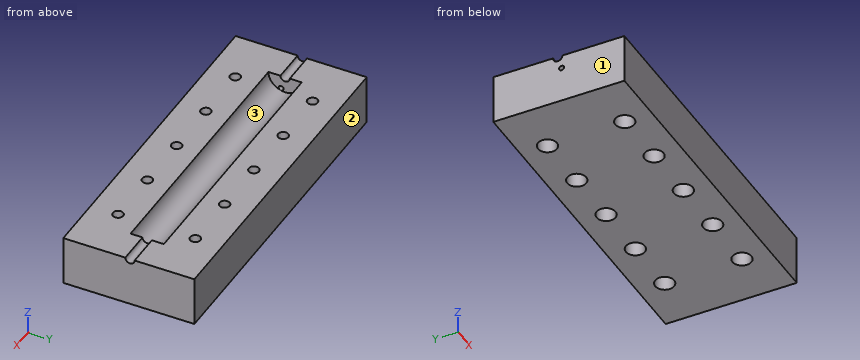
from build123d import *

# Parameters (mm, degrees)
SKIZZE2_W                            = 100
SKIZZE2_H                            = 39.364160046
AUFSATZ_LINEAR_AUSTRAGEN1_DEPTH      = 30
SCHNITT_LINEAR_AUSTRAGEN1_DEPTH      = 40
SCHNITT_LINEAR_AUSTRAGEN1_DEPTH_BACK = 40
SKIZZE10_R                           = 5
SKIZZE17_R                           = 1.4
SCHNITT_LINEAR_AUSTRAGEN2_DEPTH      = 103.710939516
SKIZZE24_R                           = 1.55
SCHNITT_LINEAR_AUSTRAGEN4_DEPTH      = 112.577493681
SKIZZE37_R                           = 0.736865544
SCHNITT_LINEAR_AUSTRAGEN9_DEPTH      = 112.577493681
SKIZZE40_R                           = 2.1
SCHNITT_LINEAR_AUSTRAGEN10_DEPTH     = 6
SKIZZE42_R                           = 0.75
SCHNITT_LINEAR_AUSTRAGEN12_DEPTH     = 10
VERRUNDUNG1_R                        = 1
SKIZZE46_R                           = 2.85
SCHNITT_LINEAR_AUSTRAGEN15_DEPTH     = 10
SCHNITT_LINEAR_START                 = -5
SCHNITT_LINEAR_AUSTRAGEN25_DEPTH     = 2.7
LINEARES_MUSTER1_COUNT               = 5
LINEARES_MUSTER1_PITCH               = 17
SPIEGELN2_COPY_1_SKETCH_R            = 2.85
SPIEGELN2_COPY_1_DEPTH               = 10
SPIEGELN2_COPY_2_SKETCH_R            = 2.85
SPIEGELN2_COPY_2_DEPTH               = 10
SPIEGELN2_COPY_3_SKETCH_R            = 2.85
SPIEGELN2_COPY_3_DEPTH               = 10
SPIEGELN2_COPY_4_SKETCH_R            = 2.85
SPIEGELN2_COPY_4_DEPTH               = 10
SPIEGELN2_START                      = -5
SPIEGELN2_COPY_5_DEPTH               = 2.7
SPIEGELN2_COPY_6_DEPTH               = 2.7
SPIEGELN2_COPY_7_DEPTH               = 2.7
SPIEGELN2_COPY_8_DEPTH               = 2.7
SKIZZE51_W                           = 15
SKIZZE51_H                           = 39.364160046
SCHNITT_LINEAR_AUSTRAGEN26_DEPTH     = 112.577493681


with BuildPart() as part:
    # Skizze2 → Aufsatz-Linear austragen1 (new body)
    with BuildSketch(Plane.XY):
        with Locations((50, 19.682080023)):
            Rectangle(SKIZZE2_W, SKIZZE2_H)
    extrude(amount=AUFSATZ_LINEAR_AUSTRAGEN1_DEPTH)

    # Skizze10 → Schnitt-Linear austragen1 (cut, two sides: drawn at the far end of the back side and taken through both)
    with BuildSketch(Plane.ZY.offset(-50).offset(-SCHNITT_LINEAR_AUSTRAGEN1_DEPTH_BACK)):
        with Locations((14.945770016, 20.027045739)):
            Circle(SKIZZE10_R)
    extrude(amount=SCHNITT_LINEAR_AUSTRAGEN1_DEPTH + SCHNITT_LINEAR_AUSTRAGEN1_DEPTH_BACK, mode=Mode.SUBTRACT)

    # Skizze17 → Schnitt-Linear austragen2 (cut, through all)
    with BuildSketch(Plane.ZY.offset(-90)):
        with Locations((14.945770016, 20.027045739)):
            Circle(SKIZZE17_R)
    schnitt_linear_austragen2 = extrude(amount=-SCHNITT_LINEAR_AUSTRAGEN2_DEPTH, mode=Mode.SUBTRACT)

    # Spiegeln1: Schnitt-Linear austragen2 across plane
    add(schnitt_linear_austragen2.mirror(Plane.ZY.offset(-50)), mode=Mode.SUBTRACT)

    # Skizze24 → Schnitt-Linear austragen4 (cut, through all)
    with BuildSketch(Plane.XY.offset(30)):
        with Locations((16, 31.364160046)):
            Circle(SKIZZE24_R)
        with Locations((33, 31.364160046)):
            Circle(SKIZZE24_R)
        with Locations((50, 31.364160046)):
            Circle(SKIZZE24_R)
        with Locations((67, 31.364160046)):
            Circle(SKIZZE24_R)
        with Locations((84, 31.364160046)):
            Circle(SKIZZE24_R)
    schnitt_linear_austragen4 = extrude(amount=-SCHNITT_LINEAR_AUSTRAGEN4_DEPTH, mode=Mode.SUBTRACT)

    # Skizze37 → Schnitt-Linear austragen9 (cut, through all)
    with BuildSketch(Plane(origin=(100, 0, 0), x_dir=(0, 0, -1), z_dir=(1, 0, 0))):
        with Locations((-18.924590299, 18.633559666)):
            Circle(SKIZZE37_R)
    extrude(amount=-SCHNITT_LINEAR_AUSTRAGEN9_DEPTH, mode=Mode.SUBTRACT)

    # Skizze40 → Schnitt-Linear austragen10 (cut)
    with BuildSketch(Plane(origin=(100, 0, 0), x_dir=(0, 0, -1), z_dir=(1, 0, 0))):
        with Locations((-18.924590299, 18.633559666)):
            Circle(SKIZZE40_R)
    extrude(amount=-SCHNITT_LINEAR_AUSTRAGEN10_DEPTH, mode=Mode.SUBTRACT)

    # Skizze42 → Schnitt-Linear austragen12 (cut)
    with BuildSketch(Plane.ZY):
        with Locations((10.86415918, 18.842582577)):
            Circle(SKIZZE42_R)
    extrude(amount=-SCHNITT_LINEAR_AUSTRAGEN12_DEPTH, mode=Mode.SUBTRACT)

    # Verrundung1
    verrundung1_edges = [part.edges().sort_by_distance(p)[0] for p in [
        (94, 18.633559666, 19.661455843),
    ]]
    fillet(verrundung1_edges, radius=VERRUNDUNG1_R)

    # Skizze46 → Schnitt-Linear austragen15 (cut)
    with BuildSketch(Plane(origin=(0, 0, 0), x_dir=(-1, 0, 0), z_dir=(0, 0, -1))):
        with Locations((-84, 31.364160046)):
            Circle(SKIZZE46_R)
    schnitt_linear_austragen15 = extrude(amount=-SCHNITT_LINEAR_AUSTRAGEN15_DEPTH, mode=Mode.SUBTRACT)

    # Skizze50 → Schnitt-Linear austragen25 (cut)
    with BuildSketch(Plane.XY.offset(30).offset(SCHNITT_LINEAR_START)):
        Polygon((81.15, 33.009608314), (81.15, 39.364160046), (86.85, 39.364160046), (86.85, 33.009608314), (86.85, 29.718711779), (84, 28.073263512), (81.15, 29.718711779), align=None)
    schnitt_linear_austragen25 = extrude(amount=-SCHNITT_LINEAR_AUSTRAGEN25_DEPTH, mode=Mode.SUBTRACT)

    # Lineares Muster1: Schnitt-Linear austragen15, Schnitt-Linear austragen25 ×5
    with Locations(*[(-i * LINEARES_MUSTER1_PITCH, 0, 0) for i in range(1, LINEARES_MUSTER1_COUNT)]):
        add(schnitt_linear_austragen15, mode=Mode.SUBTRACT)
        add(schnitt_linear_austragen25, mode=Mode.SUBTRACT)

    # Spiegeln2: Schnitt-Linear austragen15, Schnitt-Linear austragen25 across plane
    add(schnitt_linear_austragen15.mirror(Plane.ZX.offset(19.764160046)), mode=Mode.SUBTRACT)
    add(schnitt_linear_austragen25.mirror(Plane.ZX.offset(19.764160046)), mode=Mode.SUBTRACT)

    # Spiegeln2 copy 1 sketch → Spiegeln2 copy 1 (cut)
    with BuildSketch(Plane(origin=(-17, 39.528320093, 0), x_dir=(-1, 0, 0), z_dir=(0, 0, -1))):
        with Locations((-84, -31.364160046)):
            Circle(SPIEGELN2_COPY_1_SKETCH_R)
    extrude(amount=-SPIEGELN2_COPY_1_DEPTH, mode=Mode.SUBTRACT)

    # Spiegeln2 copy 2 sketch → Spiegeln2 copy 2 (cut)
    with BuildSketch(Plane(origin=(-34, 39.528320093, 0), x_dir=(-1, 0, 0), z_dir=(0, 0, -1))):
        with Locations((-84, -31.364160046)):
            Circle(SPIEGELN2_COPY_2_SKETCH_R)
    extrude(amount=-SPIEGELN2_COPY_2_DEPTH, mode=Mode.SUBTRACT)

    # Spiegeln2 copy 3 sketch → Spiegeln2 copy 3 (cut)
    with BuildSketch(Plane(origin=(-51, 39.528320093, 0), x_dir=(-1, 0, 0), z_dir=(0, 0, -1))):
        with Locations((-84, -31.364160046)):
            Circle(SPIEGELN2_COPY_3_SKETCH_R)
    extrude(amount=-SPIEGELN2_COPY_3_DEPTH, mode=Mode.SUBTRACT)

    # Spiegeln2 copy 4 sketch → Spiegeln2 copy 4 (cut)
    with BuildSketch(Plane(origin=(-68, 39.528320093, 0), x_dir=(-1, 0, 0), z_dir=(0, 0, -1))):
        with Locations((-84, -31.364160046)):
            Circle(SPIEGELN2_COPY_4_SKETCH_R)
    extrude(amount=-SPIEGELN2_COPY_4_DEPTH, mode=Mode.SUBTRACT)

    # Spiegeln2 copy 5 sketch → Spiegeln2 copy 5 (cut)
    with BuildSketch(Plane(origin=(-17, 39.528320093, 30), x_dir=(1, 0, 0), z_dir=(0, 0, 1)).offset(SPIEGELN2_START)):
        Polygon((81.15, -33.009608314), (81.15, -39.364160046), (86.85, -39.364160046), (86.85, -33.009608314), (86.85, -29.718711779), (84, -28.073263512), (81.15, -29.718711779), align=None)
    extrude(amount=-SPIEGELN2_COPY_5_DEPTH, mode=Mode.SUBTRACT)

    # Spiegeln2 copy 6 sketch → Spiegeln2 copy 6 (cut)
    with BuildSketch(Plane(origin=(-34, 39.528320093, 30), x_dir=(1, 0, 0), z_dir=(0, 0, 1)).offset(SPIEGELN2_START)):
        Polygon((81.15, -33.009608314), (81.15, -39.364160046), (86.85, -39.364160046), (86.85, -33.009608314), (86.85, -29.718711779), (84, -28.073263512), (81.15, -29.718711779), align=None)
    extrude(amount=-SPIEGELN2_COPY_6_DEPTH, mode=Mode.SUBTRACT)

    # Spiegeln2 copy 7 sketch → Spiegeln2 copy 7 (cut)
    with BuildSketch(Plane(origin=(-51, 39.528320093, 30), x_dir=(1, 0, 0), z_dir=(0, 0, 1)).offset(SPIEGELN2_START)):
        Polygon((81.15, -33.009608314), (81.15, -39.364160046), (86.85, -39.364160046), (86.85, -33.009608314), (86.85, -29.718711779), (84, -28.073263512), (81.15, -29.718711779), align=None)
    extrude(amount=-SPIEGELN2_COPY_7_DEPTH, mode=Mode.SUBTRACT)

    # Spiegeln2 copy 8 sketch → Spiegeln2 copy 8 (cut)
    with BuildSketch(Plane(origin=(-68, 39.528320093, 30), x_dir=(1, 0, 0), z_dir=(0, 0, 1)).offset(SPIEGELN2_START)):
        Polygon((81.15, -33.009608314), (81.15, -39.364160046), (86.85, -39.364160046), (86.85, -33.009608314), (86.85, -29.718711779), (84, -28.073263512), (81.15, -29.718711779), align=None)
    extrude(amount=-SPIEGELN2_COPY_8_DEPTH, mode=Mode.SUBTRACT)

    # Spiegeln3: Schnitt-Linear austragen4 across plane
    add(schnitt_linear_austragen4.mirror(Plane.ZX.offset(19.764160046)), mode=Mode.SUBTRACT)

    # Skizze51 → Schnitt-Linear austragen26 (cut, through all)
    with BuildSketch(Plane.ZY):
        with Locations((22.5, 19.682080023)):
            Rectangle(SKIZZE51_W, SKIZZE51_H)
    extrude(amount=-SCHNITT_LINEAR_AUSTRAGEN26_DEPTH, mode=Mode.SUBTRACT)


solid = part.part
The model under review builds one solid part; all positions refer to its coordinate system, in mm. Face numbers are marked on the shaded views. Round coordinates to 2 decimals unless told otherwise and drop trailing zeros. Loops run counter-clockwise (first coordinate to the right, second up) from the corner with the lowest first, then second, coordinate; pieces in that order, holes last. Notation, with made-up numbers: M -6,-2 L 3,-2 A21 cw 3,10 Z; hole C -6,-39.75 d7. An arc over 180 degrees is marked long. Answer as a JSON object with one key per item and string values.
Item 1: We need section A-A, the plane x = 16. State the section outline as (y, z) points, and give its area (3 significant figures).
Check sheet entries:
{"outline": "M 0,0 L 5.31,0 L 5.31,10 L 6.61,10 L 6.61,15 L 0,15 Z; M 9.71,10 L 11.01,10 L 11.01,0 L 28.51,0 L 28.51,10 L 29.81,10 L 29.81,15 L 25.03,15 A5 cw long 15.03,15 L 9.71,15 Z; M 32.91,10 L 34.21,10 L 34.21,0 L 39.36,0 L 39.36,15 L 32.91,15 Z", "area": "406 mm2"}
Item 2: For line 1 along Y through (x, z) = (84, 3); line 2 along Y through (x, z) = (67, 12.5); line 3 along Y through (x, z) = (66.5, 13), list the stretches that pass through material, from the lowest coordinate up.
Check sheet entries:
{"line 1": "0 to 5.31, 11.01 to 28.51, 34.21 to 39.36", "line 2": "0 to 6.61, 9.71 to 15.67, 24.39 to 29.81, 32.91 to 39.36", "line 3": "0 to 6.7, 9.63 to 15.42, 24.63 to 29.9, 32.83 to 39.36"}
Item 3: We need section C-C, the plane y = 23.5. State the section outline as (x, z) points, and give its area (3 significant figures).
Check sheet entries:
{"outline": "M 0,0 L 100,0 L 100,15 L 90,15 L 90,11.35 L 10,11.35 L 10,15 L 0,15 Z", "area": "1,210 mm2"}
Item 4: The part is to be moulded in two halves that separate along Y. For the marked faces 1, 2 and 3, say which applies: +Y half, -Y half, draft (parallel to the pull), parting line (faces both ways), or undercut.
Check sheet entries:
{"face 1": "draft", "face 2": "+Y half", "face 3": "undercut"}
Item 5: We need section B-B, the plane z = 7.25. State how many separate pieces and enclosed holes the cut face has, and give its area (3 significant figures).
Check sheet entries:
{"separate pieces": "1", "enclosed holes": "10", "area": "3,680 mm2"}
Item 6: Clearance check with flat-ended pins moving along their axes: P1, Ø5, axis at x = 50, y = 8.16, coming from the -Z side; P2, Ø2.5, axis at x = 16, y = 31.36, coming from the +Z side; P3, Ø4, axis at y = 22, z = 13.5, coming from the -X side. State where each tip first meets the part, or that it passes through.
Check sheet entries:
{"P1": "z = 10", "P2": "through", "P3": "x = 0"}
